```python
from build123d import *

# Parameters (mm, degrees)
F1_DEPTH = 6.35
F3_DEPTH = 25.4
F4_R     = 15.875
F4_R_2   = 22.225
F4_R_3   = 41.275
F4_R_4   = 28.575
F4_R_5   = 34.925
F5_DEPTH = 25.4


with BuildPart() as f1:
    # F0 (on Front) → F1 (new body)
    with BuildSketch(Plane.XZ):
        Polygon((-120.65, 342.9), (-120.65, 0), (0, 0), (0, 342.9), (146.05, 762), (12.7, 762), align=None)
        Polygon((12.7, 850.9), (12.7, 762), (146.05, 762), (247.65, 762), (247.65, 850.9), align=None)
    extrude(amount=F1_DEPTH)

    # F2 (on face) → F3 (cut)
    with BuildSketch(Plane.XZ.offset(6.35)):
        Polygon((247.65, 850.9), (190.5, 850.9), (247.65, 800.1), align=None)
    extrude(amount=-F3_DEPTH, mode=Mode.SUBTRACT)

    # F4 (on face) → F5 (cut)
    with BuildSketch(Plane.XZ.offset(6.35)):
        with Locations((-60.325, 342.9)):
            Circle(F4_R)
        with Locations((-30.1625, 433.3875)):
            Circle(F4_R_2)
        with Locations((60.325, 704.85)):
            Circle(F4_R_3)
        Polygon((186.552938, 838.2), (186.164132, 837.762077), (214.640432, 812.44981), align=None)
        Polygon((234.95, 794.396861), (233.624632, 795.574966), (215.09097, 774.7), (234.95, 774.7), align=None)
        with Locations((0, 523.875)):
            Circle(F4_R_4)
        with Locations((30.1625, 614.3625)):
            Circle(F4_R_5)
        Polygon((67.670581, 838.2), (25.4, 838.2), (25.4, 790.589499), align=None)
        Polygon((152.58655, 838.2), (101.636968, 838.2), (45.25903, 774.7), (96.208612, 774.7), align=None)
        Polygon((214.640432, 812.44981), (186.164132, 837.762077), (130.175, 774.7), (181.124582, 774.7), align=None)
        with Locations((-60.325, 247.523)):
            Circle(F4_R_2)
        with Locations((-60.325, 152.146)):
            Circle(F4_R_4)
        with Locations((-60.325, 56.769)):
            Circle(F4_R_5)
    extrude(amount=-F5_DEPTH, mode=Mode.SUBTRACT)


solid = f1.part
```
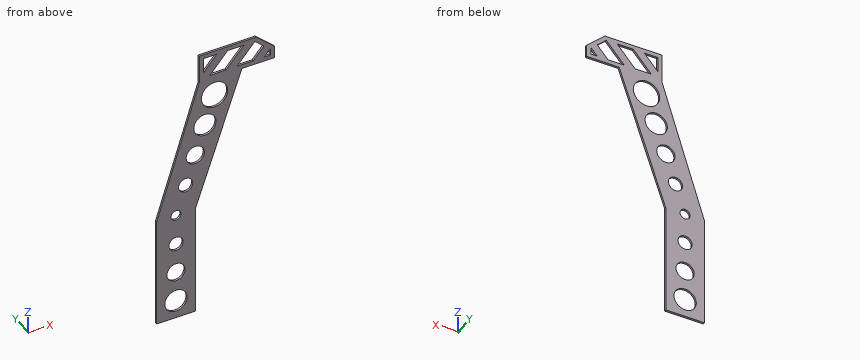
Could you check a few things on this model? Use its own coordinates, in mm. Round coordinates to 2 decimals unless told otherwise and drop trailing zeros. Loops run counter-clockwise (first coordinate to the right, second up) from the corner with the lowest first, then second, coordinate; pieces in that order, holes last. Notation, with made-up numbers: (9, 72) - (44, 72) arc R28 cw to (44, 111) - close; hole circle Ø2 at (39.25, 19.25). An arc over 180 degrees is marked (long way). Answer as CSV lines item,"result".
1. Please list where these lines run through material, in increasing order: line 1 along X through (y, z) = (-0.75, 248); line 2 along Z through (x, y) = (223, -3.75); line 3 along X through (y, z) = (-3.75, 334.5). Write a range as [from, to].
Filled in:
line 1,"x = [-120.65, -82.54], [-38.11, 0]"
line 2,"z = [762, 774.7], [783.61, 822.01]"
line 3,"x = [-120.65, -73.8], [-46.85, 0]"
2. For pin 1 Ø1.5 at (y, z) = (-4.5, 645.5) entering from +X; pin 2 Ø3 at (y, z) = (-2.5, 805.5) entering from +X; pin 3 Ø12 at (x, z) = (-47.5, 393.5) entering from +Y; pin 4 Ø1.9 at (y, z) = (-3, 140) entering from +X, each with a flat end and sliding along its axis, tell me the tip position at first contact or that it passes through.
Filled in:
pin 1,"stops at x = 105.71"
pin 2,"stops at x = 243.26"
pin 3,"stops at y = 0"
pin 4,"stops at x = 0"
3. I want a section at C-C on y = -4.25. Count the separate pieces of the cut face and the enclosed holes in it, then the cut area to 3 significant figures.
Filled in:
separate pieces,"1"
enclosed holes,"12"
area,"84,900 mm^2"
4. I want a section at A-A on z = 424. List the corners of the cut face in (x, y) for me.
Filled in:
outline,"(-94.85, -6.35) - (-50.31, -6.35) - (-50.31, 0) - (-94.85, 0) - close; (-10.02, -6.35) - (28.26, -6.35) - (28.26, 0) - (-10.02, 0) - close"
5. I want a section at B-B on x = 122.5. List the corners of the cut face in (y, z) for me.
Filled in:
outline,"(-6.35, 694.42) - (0, 694.42) - (0, 804.31) - (-6.35, 804.31) - close; (-6.35, 838.2) - (0, 838.2) - (0, 850.9) - (-6.35, 850.9) - close"
6. I want a section at D-D on z = 99.5. List the corners of the cut face in (x, y) for me, then the cut area to 3 significant figures.
Filled in:
outline,"(-120.65, -6.35) - (0, -6.35) - (0, 0) - (-120.65, 0) - close"
area,"766 mm^2"
